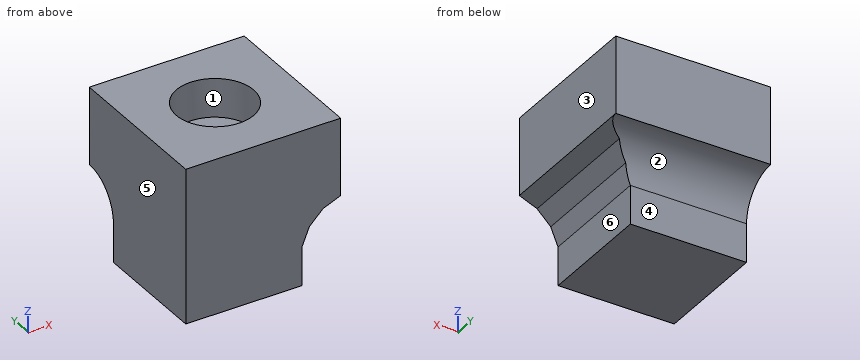
```python
from build123d import *

# Parameters (mm, degrees)
F0_W          = 20
F0_H          = 20
F1_DEPTH      = 20
F3_DEPTH      = 10.001
F3_DEPTH_BACK = 10.001
F5_DEPTH      = 10.001
F5_DEPTH_BACK = 10.001
F6_R          = 5
F7_DEPTH      = 5


with BuildPart() as f1:
    # F0 (on Top) → F1 (new body)
    with BuildSketch(Plane.XY):
        Rectangle(F0_W, F0_H)
    extrude(amount=F1_DEPTH)

    # F2 (on Front) → F3 (cut, two sides)
    with BuildSketch(Plane.XZ) as f3_sk:
        Polygon((5, 5), (5, 0), (10, 0), (10, 10), (7.7059805007, 9.0497860111), (5.9502139889, 7.2940194993), align=None)
    extrude(amount=-F3_DEPTH, mode=Mode.SUBTRACT)
    extrude(f3_sk.sketch, amount=F3_DEPTH_BACK, mode=Mode.SUBTRACT)

    # F4 (on Right) → F5 (cut, two sides)
    with BuildSketch(Plane.YZ) as f5_sk:
        with BuildLine():
            Line((5, 5), (5, 0))
            Line((5, 0), (10, 0))
            Line((10, 0), (10, 10))
            ThreePointArc((10, 10), (6.4644660941, 8.5355339059), (5, 5))
        make_face()
    extrude(amount=-F5_DEPTH, mode=Mode.SUBTRACT)
    extrude(f5_sk.sketch, amount=F5_DEPTH_BACK, mode=Mode.SUBTRACT)

    # F6 (on face) → F7 (cut)
    with BuildSketch(Plane.XY.offset(20)):
        Circle(F6_R)
    extrude(amount=-F7_DEPTH, mode=Mode.SUBTRACT)


solid = f1.part
```
Geometry: final body of the model. Coordinates: model frame, mm. Face numbers are marked on the shaded views. A direction names the side the tool comes from. Coordinates: 2 decimals unless noted, no trailing zeros. Write each loop counter-clockwise with the first axis right and the second up, starting at its lowest first coordinate (ties: lowest second). Pieces come first, ordered by that corner, then holes. Notation, with made-up numbers: M -0.75,20 L 22.25,20 A12 ccw 22.25,39 Z; hole C 60.5,-37 d3. An arc over 180 degrees is marked long. Answer as CSV lines item,"result". Start each with the question number.
Q1. Cut plane C-C on z = 3. Return the cut outline in (x, y), then the cut area to 3 significant figures.
Q2. Cut plane B-B on y = 0. Return the cut outline in (x, z), then the cut area to 3 significant figures.
Q3. Mould query, pull axis Y, two halves, no side actions, for the marked faces 1, 2 and 3. Classes: released by +Y, released by -Y, zero draft, split by the parting line, or undercut.
Q4. Pin query (flat end, axial travel): P1, Ø11, axis at x = 1, y = 2, coming from the +Z side; P2, Ø5.5, axis at y = -2, z = 2.5, coming from the +X side; P3, Ø6, axis at x = 8, y = 5.5, coming from the -Z side; P4, Ø4, axis at x = -2.5, z = 2, coming from the +Y side. Return the tip coordinate at first contact, or that it passes through.
Q5. Cut plane D-D on y = -3.5. Return the cut outline in (x, z), then the cut area to 3 significant figures.
Q6. Cut plane A-A on x = 0. Return the cut outline in (y, z), then the cut area to 3 significant figures.
Q7. Reachability of the marked faces 4, 5 and 6 from +Z, -Z, +X, -X, +Y, -Y: full face, straight path, thin tool, end or side. Return the list, or none.
Q8. Line query: line 1 (Y direction, x = 0, z = 17.5); line 2 (Z direction, x = -3.25, y = -3.5); line 3 (X direction, y = 3.25, z = 17.5). Output: solid intervals per line, ascending. Write a range as from..to.
Findings below:
1,outline,"M -10,-10 L 5,-10 L 5,5 L -10,5 Z"
1,area,"225 mm2"
2,outline,"M -10,0 L 5,0 L 5,5 L 5.95,7.29 L 7.71,9.05 L 10,10 L 10,20 L 5,20 L 5,15 L -5,15 L -5,20 L -10,20 Z"
2,area,"308 mm2"
3,face 1,"undercut"
3,face 2,"released by +Y"
3,face 3,"zero draft"
4,P1,"stops at z = 20"
4,P2,"stops at x = 5.1"
4,P3,"stops at z = 5.1"
4,P4,"stops at y = 5"
5,outline,"M -10,0 L 5,0 L 5,5 L 5.95,7.29 L 7.71,9.05 L 10,10 L 10,20 L 3.57,20 L 3.57,15 L -3.57,15 L -3.57,20 L -10,20 Z"
5,area,"322 mm2"
6,outline,"M -10,0 L 5,0 L 5,5 A5 cw 10,10 L 10,20 L 5,20 L 5,15 L -5,15 L -5,20 L -10,20 Z"
6,area,"305 mm2"
7,face 4,"-Z, +X, -X, +Y"
7,face 5,"+Z, -Z, -X, +Y, -Y"
7,face 6,"-Z, +X, +Y, -Y"
8,line 1,"y = -10..-5, 5..10"
8,line 2,"z = 0..15"
8,line 3,"x = -10..-3.8, 3.8..10"
